from build123d import *

# Parameters (mm, degrees)
SKETCH1_R               = 1.6
BOSS_EXTRUDE1_DEPTH     = 8
CUT_EXTRUDE1_DEPTH      = 68.432753975
CUT_EXTRUDE1_DEPTH_BACK = 68.432753975
SKETCH2_R               = 1.75
SKETCH2_R_2             = 1.6
FILLET1_R               = 10


with BuildPart() as part:
    # Sketch1 → Boss-Extrude1 (new body)
    with BuildSketch(Plane(origin=(0, 0, 0), x_dir=(1, 0, 0), z_dir=(0, 1, 0))):
        with BuildLine():
            Line((-6.523802572, 1), (-66.523802572, 1))
            Line((-66.523802572, 1), (-66.523802572, -1))
            Line((-66.523802572, -1), (-6.523802572, -1))
            ThreePointArc((-6.523802572, -1), (0, -6.6), (6.523802572, -1))
            ThreePointArc((6.523802572, -1), (6.6, 0), (6.523802572, 1))
            ThreePointArc((6.523802572, 1), (0, 6.6), (-6.523802572, 1))
        make_face()
        with Locations(Location((0, 0, 0), (0, 0, 270))):
            Circle(SKETCH1_R, mode=Mode.SUBTRACT)
    extrude(amount=BOSS_EXTRUDE1_DEPTH)

    # Sketch2 → Cut-Extrude1 (cut, two sides: drawn at the far end of the back side and taken through both)
    with BuildSketch(Plane.XY.offset(1).offset(-CUT_EXTRUDE1_DEPTH_BACK)):
        with BuildLine():
            Line((-66.523802572, 8), (-66.523802572, 4))
            ThreePointArc((-66.523802572, 4), (-65.352229697, 6.828427125), (-62.523802572, 8))
            Line((-62.523802572, 8), (-66.523802572, 8))
        make_face()
        with BuildLine():
            Line((-66.523802572, 4), (-66.523802572, 0))
            Line((-66.523802572, 0), (-62.523802572, 0))
            ThreePointArc((-62.523802572, 0), (-65.352229697, 1.171572875), (-66.523802572, 4))
        make_face()
        with Locations((-62.523802572, 4)):
            Circle(SKETCH2_R)
        with Locations((0, 4)):
            Circle(SKETCH2_R_2)
    extrude(amount=CUT_EXTRUDE1_DEPTH + CUT_EXTRUDE1_DEPTH_BACK, mode=Mode.SUBTRACT)

    # Fillet1
    fillet1_edges = [part.edges().sort_by_distance(p)[0] for p in [
        (-6.523802572, 4, 1),
        (-6.523802572, 4, -1),
    ]]
    fillet(fillet1_edges, radius=FILLET1_R)


solid = part.part
Build history of the part. All positions in model axes, mm. A direction names the side the tool comes from. Round coordinates to 2 decimals unless told otherwise and drop trailing zeros. Write each loop counter-clockwise with the first axis right and the second up, starting at its lowest first coordinate (ties: lowest second). Pieces come first, ordered by that corner, then holes. Notation, with made-up numbers: (68.25, 88) -> (123.25, 88) arc R25 ccw to (123.25, 114) -> close; hole circle Ø3 at (80.5, 51.25). An arc over 180 degrees is marked (long way). Write item = value, one per line.
(1) Flat gauge pins, fed straight in: pin 1 (3.5 mm diameter, centred on x = 0, y = 4, fed in from -Z); pin 2 (2.5 mm diameter, centred on x = -52, y = 4, fed in from +Z); pin 3 (2.5 mm diameter, centred on x = 0, y = 4, fed in from -Z); pin 4 (1.5 mm diameter, centred on y = 6, z = -1, fed in from +X). Where does each tip first touch, or does it go through?
Answer:
pin_1 = -6.6
pin_2 = 1
pin_3 = through
pin_4 = 6.6
(2) Band-saw the part on A-A (y = 5). Give the cut face in (x, z).
Answer:
outline = (-66.4, -1) -> (-63.96, -1) -> (-63.96, 1) -> (-66.4, 1) -> close; (-61.09, -1) -> (-12.43, -1) arc R10 cw to (-4.94, -4.37) arc R6.6 ccw to (-1.25, -6.48) -> (-1.25, -1) arc R1.6 cw to (-1.25, 1) -> (-1.25, 6.48) arc R6.6 ccw to (-4.94, 4.37) arc R10 cw to (-12.43, 1) -> (-61.09, 1) -> close; (1.25, -6.48) arc R6.6 ccw to (1.25, 6.48) -> (1.25, 1) arc R1.6 cw to (1.25, -1) -> close
(3) Band-saw the part on C-C (x = -22.5). Give the cut face in (y, z), then the cut area to 3 significant figures.
Answer:
outline = (0, -1) -> (8, -1) -> (8, 1) -> (0, 1) -> close
area = 16.0 mm2
(4) Probe L1, parallel to Y at x = 0, z = 3.5; L2, parallel to Z at x = 0, y = 1.35; L3, parallel to Z at x = -32, y = 4.75. List the from-to ranges inside material, lowest first.
Answer:
L1 = 0 to 2.4, 5.6 to 8
L2 = -6.6 to -1.6, 1.6 to 6.6
L3 = -1 to 1
(5) Two-plate mould, pull along X, no slides. Class faces 4 (the face through (-15, 0, 0)), 5 (the face through (-60.907, 3.33, -0.014)), 6 (the face through (-8.38, 4.06, -1.86)): pulls with the +X half, pulls with the -X half, needs draft (parallel to the pull), parting line crosses it, or undercut.
Answer:
face_4 = needs draft
face_5 = undercut
face_6 = pulls with the -X half
(6) Tool access for faces 1 (the face through (-40, 4, 1)), 2 (the face through (-1.27, 3.03, 3.99)), 3 (the face through (-39, 4, -1)): list every direction of +Z, -Z, +X, -X, +Y, -Y with a clear straight run to the whole face (end or side of a thin tool).
Answer:
face_1 = +Z, -X, +Y, -Y
face_2 = +Z, -Z
face_3 = -Z, -X, +Y, -Y
(7) Band-saw the part on B-B (z = -3). Give the cut face in (x, y), then the cut area to 3 significant figures.
Answer:
outline = (-6.43, 0) -> (5.88, 0) -> (5.88, 8) -> (-6.43, 8) -> close; hole circle Ø3.2 at (0, 4)
area = 90.4 mm2
